from build123d import *
from build123d.topology import SkipClean

# Parameters (mm, degrees)
SKETCH1_R                            = 19.5
SKETCH1_R_2                          = 14.75
BOSS_EXTRUDE1_DEPTH                  = 57
SKETCH2_R                            = 3
BOSS_EXTRUDE2_DEPTH                  = 2
BOSS_EXTRUDE2_DIRECTION_2_REACH      = 73.765
BOSS_EXTRUDE2_DIRECTION_2_END_RADIUS = 19.5
SKETCH3_R                            = 3
BOSS_EXTRUDE4_DEPTH                  = 2
BOSS_EXTRUDE4_DIRECTION_2_REACH      = 74.871
BOSS_EXTRUDE4_DIRECTION_2_END_RADIUS = 19.5
FILLET3_R                            = 1


with BuildPart() as part:
    # Sketch1 → Boss-Extrude1 (new, symmetric)
    with BuildSketch(Plane(origin=(0, 0, 0), x_dir=(1, 0, 0), z_dir=(0, 1, 0))):
        with Locations(Location((0, 0, 0), (0, 0, 90))):
            Circle(SKETCH1_R)
        with Locations(Location((0, 0, 0), (0, 0, 90))):
            Circle(SKETCH1_R_2, mode=Mode.SUBTRACT)
    extrude(amount=BOSS_EXTRUDE1_DEPTH, both=True)


with BuildPart() as body_2:
    # Sketch2 → Boss-Extrude2 (new body)
    with BuildSketch(Plane(origin=(19.5, 0, 0), x_dir=(0, 0, -1), z_dir=(1, 0, 0))):
        with Locations((0, -45)):
            Circle(SKETCH2_R)
        Circle(SKETCH2_R)
    extrude(amount=BOSS_EXTRUDE2_DEPTH)

    # Boss-Extrude2 direction 2: up to this cylinder (the profile starts outside it)
    with SkipClean():  # the faces are left unmerged after this step: merging them gives an invalid solid
        boss_extrude2_direction_2_end = Plane(origin=(0, -22.5, 0), z_dir=(0, -1, 0)) * Cylinder(BOSS_EXTRUDE2_DIRECTION_2_END_RADIUS, 232.53, mode=Mode.PRIVATE)
        # Sketch2 → Boss-Extrude2 direction 2 (add, up to the surface)
        with BuildSketch(Plane(origin=(19.5, 0, 0), x_dir=(0, 0, -1), z_dir=(1, 0, 0)), mode=Mode.PRIVATE) as boss_extrude2_direction_2_sk1:
            with Locations((0, -45)):
                Circle(SKETCH2_R)
        boss_extrude2_direction_2_tool1 = extrude(boss_extrude2_direction_2_sk1.sketch, amount=-BOSS_EXTRUDE2_DIRECTION_2_REACH, mode=Mode.PRIVATE) - boss_extrude2_direction_2_end
        add(boss_extrude2_direction_2_tool1.solids().sort_by_distance((19.5, -45, 0))[0])
        add(boss_extrude2_direction_2_tool1.solids().sort_by_distance((19.5, -45, 0))[1])
        # Sketch2 → Boss-Extrude2 direction 2 (add, up to the surface)
        with BuildSketch(Plane(origin=(19.5, 0, 0), x_dir=(0, 0, -1), z_dir=(1, 0, 0)), mode=Mode.PRIVATE) as boss_extrude2_direction_2_sk2:
            Circle(SKETCH2_R)
        boss_extrude2_direction_2_tool2 = extrude(boss_extrude2_direction_2_sk2.sketch, amount=-BOSS_EXTRUDE2_DIRECTION_2_REACH, mode=Mode.PRIVATE) - boss_extrude2_direction_2_end
        add(boss_extrude2_direction_2_tool2.solids().sort_by_distance((19.5, 0, 0))[0])
        add(boss_extrude2_direction_2_tool2.solids().sort_by_distance((19.5, 0, 0))[1])


with BuildPart() as body_3:
    # Sketch3 → Boss-Extrude4 (new body)
    with BuildSketch(Plane.ZY.offset(19.5)):
        Circle(SKETCH3_R)
    extrude(amount=BOSS_EXTRUDE4_DEPTH)

    # Boss-Extrude4 direction 2: up to this cylinder (the profile starts outside it)
    with SkipClean():  # the faces are left unmerged after this step: merging them gives an invalid solid
        boss_extrude4_direction_2_end = Plane(origin=(0, 0, 0), z_dir=(0, -1, 0)) * Cylinder(BOSS_EXTRUDE4_DIRECTION_2_END_RADIUS, 189.742, mode=Mode.PRIVATE)
        # Sketch3 → Boss-Extrude4 direction 2 (add, up to the surface)
        with BuildSketch(Plane.ZY.offset(19.5), mode=Mode.PRIVATE) as boss_extrude4_direction_2_sk1:
            Circle(SKETCH3_R)
        boss_extrude4_direction_2_tool1 = extrude(boss_extrude4_direction_2_sk1.sketch, amount=-BOSS_EXTRUDE4_DIRECTION_2_REACH, mode=Mode.PRIVATE) - boss_extrude4_direction_2_end
        add(boss_extrude4_direction_2_tool1.solids().sort_by_distance((-19.5, 0, 0))[0])
        add(boss_extrude4_direction_2_tool1.solids().sort_by_distance((-19.5, 0, 0))[1])


with BuildPart() as body_2_1:
    add(body_2.part)

    # Combine1: union part, body 3
    add(part.part)
    add(body_3.part)

    # Fillet3
    fillet3_edges = [body_2_1.edges().sort_by_distance(p)[0] for p in [
        (19.267848866, -45, 3.000000015),
        (19.267848866, 0, 3.000000015),
        (-19.267848866, 0, -3.000000015),
    ]]
    fillet(fillet3_edges, radius=FILLET3_R)


solid = body_2_1.part
Could you check a few things on this model? Use its own coordinates, in mm. A direction names the side the tool comes from. Coordinates: 2 decimals unless noted, no trailing zeros. Loops run counter-clockwise (first coordinate to the right, second up) from the corner with the lowest first, then second, coordinate; pieces in that order, holes last.
1. For P1, Ø10, axis at x = -12.5, y = -43.5, coming from the +Z side; P2, Ø4, axis at y = -14, z = -3, coming from the +X side; P3, Ø4, axis at x = 15.5, y = -11, coming from the +Z side; P4, Ø4, axis at x = -7.5, z = -10, coming from the -Y side, each with a flat end and sliding along its axis, tell me the tip position at first contact or that it passes through.
2. Imagine slicing it at C-C (y = 30). Please give me the cut outline in (x, z).
3. We'd pull the mould along Z, two halves only. Please class faces 1 (the face through (-4.43, -0.8, -14.07)), 2 (the face through (-21.5, 0, 0)), 3 (the face through (19.036, 0.798, 4.227)): released by +Z, released by -Z, zero draft, split by the parting line, or undercut.
4. For faces 4 (the face through (-20.95, -1.15, 2.77)), 5 (the face through (21.5, 0, 0)), 6 (the face through (20.95, 0.9, -2.86)), which set-ups out of +Z, -Z, +X, -X, +Y, -Y let a thin tool reach every point of the face, with its end or its side?
5. Imagine slicing it at B-B (z = -9). Please give me the cut outline in (x, y), and give its area (3 significant figures).
6. Imagine slicing it at D-D (x = -17.5). Please give me the cut outline in (y, z).
7. Imagine slicing it at A-A (x = 0). Please give me the cut outline in (y, z), and give its area (3 significant figures).
8. I need wall thicknesses on L1, parallel to X at y = 2.5, z = 0; L2, parallel to X at y = -19.5, z = 0; L3, parallel to Z at x = -0.5, y = -12.5. Which ranges of each line are inside material? Lowest first, please.
Computed values:
1. P1: stops at z = 18
1. P2: stops at x = 19.47
1. P3: stops at z = 14.07
1. P4: passes through
2. outline: circle Ø39 at (0, 0); hole circle Ø29.5 at (0, 0)
3. face 1: undercut
3. face 2: zero draft
3. face 3: split by the parting line
4. face 4: -X
4. face 5: +Z, -Z, +X, +Y, -Y
4. face 6: +X
5. outline: (-17.3, -57) - (-11.69, -57) - (-11.69, 57) - (-17.3, 57) - close; (11.69, -57) - (17.3, -57) - (17.3, 57) - (11.69, 57) - close
5. area: 1,280 mm2
6. outline: (-57, -8.6) - (57, -8.6) - (57, 8.6) - (-57, 8.6) - close
7. outline: (-57, -19.5) - (57, -19.5) - (57, -14.75) - (-57, -14.75) - close; (-57, 14.75) - (57, 14.75) - (57, 19.5) - (-57, 19.5) - close
7. area: 1,080 mm2
8. L1: x = -21.5 to -14.75, 14.75 to 21.5
8. L2: x = -19.5 to -14.75, 14.75 to 19.5
8. L3: z = -19.49 to -14.74, 14.74 to 19.49
